Source: CAD feature listing. Evaluate the final solid. Frame: model axes, mm. A direction names the side the tool comes from. Give positions to 0.01 mm unless a question says otherwise; leave off trailing zeros. Loops run counter-clockwise (first coordinate to the right, second up) from the corner with the lowest first, then second, coordinate; pieces in that order, holes last. Notation, with made-up numbers: (8.25, -32) - (67.25, -32) arc R23 cw to (67.25, -14) - close; hole circle Ø5 at (79, -24). An arc over 180 degrees is marked (long way). Write each question's results on one line, items separated by ' | '. Start each with the question number.
(1) Reachability of faces 1 (the cylindrical face through (0.333, -1.463, 2.535)), 2 (the flat face through (0, 0, 5)) from +Z, -Z, +X, -X, +Y, -Y: full face, straight path, thin tool, end or side. Return the list, or none.
(2) Cut plane D-D on x = 0.25. Return the cut outline in (y, z), then the cut area to 3 significant figures.
(3) Cut plane C-C on x = 2.5. Return the cut outline in (y, z), then the cut area to 3 significant figures.
(4) Contact query for flat-ended pins moving along their axis: pin 1 (2 mm diameter, centred on x = 1.5, z = 2, fed in from -Y); pin 2 (3 mm diameter, centred on y = 3.5, z = 1.5, fed in from +X); pin 3 (2 mm diameter, centred on x = 5, z = 0.5, fed in from -Y). Output: stop coordinate, or through.
(5) Material intervals for line 1 along X through (y, z) = (-4, 3.2); line 2 along X through (y, z) = (4, 3.7); line 3 along Y through (x, z) = (-4.5, 2.35), sorted ascending. Write a range as [from, to].
(6) Cut plane B-B on y = -1.75. Return the cut outline in (x, z), then the cut area to 3 significant figures.
(7) Cut plane A-A on z = 0.45. Return the cut outline in (x, y).
(8) Pull-direction query (Y, two-part tool) for faces 3 (the flat face through (0, 0, 0)), 4 (the cylindrical face through (-1.46, -6.59, 2.46)), 5 (the flat face through (0, 4, 3)); classes: pulls with the +Y half, pulls with the -Y half, needs draft (parallel to the pull), parting line crosses it, or undercut.
from build123d import *

# Parameters (mm, degrees)
F0_R     = 6.75
F1_DEPTH = 5
F3_DEPTH = 25


# Not quite as in the source:
# - a feature names something its author has since deleted; it is built from what else it names


with BuildPart() as f1:
    # F0 (on Top) → F1 (new body)
    with BuildSketch(Plane.XY):
        Circle(F0_R)
    extrude(amount=F1_DEPTH)

    # F2 (on face) → F3 (cut)
    with BuildSketch(Plane.XY.offset(5)):
        with BuildLine():
            Line((1.0970305524, 1.0229975401), (4.02115299, 3.7497858268))
            ThreePointArc((4.02115299, 3.7497858268), (2.192415253, 5.04220988), (0, 5.4982329084))
            Line((0, 5.4982329084), (0, 1.5))
            ThreePointArc((0, 1.5), (0.5981236034, 1.3755901116), (1.0970305524, 1.0229975401))
        make_face()
        with BuildLine():
            Line((-0.6339273926, 1.3594616806), (-2.3236536344, 4.9830912999))
            ThreePointArc((-2.3236536344, 4.9830912999), (-4.117932991, 3.6432393549), (-5.2291302357, 1.6990474077))
            Line((-5.2291302357, 1.6990474077), (-1.4265847744, 0.4635254916))
            ThreePointArc((-1.4265847744, 0.4635254916), (-1.1234335812, 0.9939300723), (-0.6339273926, 1.3594616806))
        make_face()
        with BuildLine():
            ThreePointArc((-5.4572499141, -0.6700660344), (-4.7374378048, -2.7905641295), (-3.2317802172, -4.448163862))
            Line((-3.2317802172, -4.448163862), (-0.8816778784, -1.2135254916))
            ThreePointArc((-0.8816778784, -1.2135254916), (-1.2924437407, -0.7613075444), (-1.4888192275, -0.1828040151))
            Line((-1.4888192275, -0.1828040151), (-5.4572499141, -0.6700660344))
        make_face()
        with BuildLine():
            ThreePointArc((-1.0491122976, -5.3972148839), (1.190035408, -5.3679028347), (3.2317802172, -4.448163862))
            Line((3.2317802172, -4.448163862), (0.8816778784, -1.2135254916))
            ThreePointArc((0.8816778784, -1.2135254916), (0.3246594209, -1.4644440107), (-0.2862134931, -1.4724407752))
            Line((-0.2862134931, -1.4724407752), (-1.0491122976, -5.3972148839))
        make_face()
        with BuildLine():
            ThreePointArc((4.8088628562, -2.6655962084), (5.3231012166, -1.3766475779), (5.4982329084, 0))
            ThreePointArc((5.4982329084, 0), (5.4305405375, 0.8601131237), (5.2291302357, 1.6990474077))
            Line((5.2291302357, 1.6990474077), (1.4265847744, 0.4635254916))
            ThreePointArc((1.4265847744, 0.4635254916), (1.4815325109, 0.2346516976), (1.5, 0))
            ThreePointArc((1.5, 0), (1.4522214606, -0.3755700061), (1.3119295607, -0.7272144304))
            Line((1.3119295607, -0.7272144304), (4.8088628562, -2.6655962084))
        make_face()
    extrude(amount=-F3_DEPTH, mode=Mode.SUBTRACT)


solid = f1.part
Ans:
1) face 1: +Z, -Z | face 2: +Z, +X, -X, +Y, -Y
2) outline: (-6.75, 0) - (-5.49, 0) - (-5.49, 5) - (-6.75, 5) - close; (-1.48, 0) - (1.48, 0) - (1.48, 5) - (-1.48, 5) - close; (5.49, 0) - (6.75, 0) - (6.75, 5) - (5.49, 5) - close | area: 27.3 mm^2
3) outline: (-6.27, 0) - (-4.9, 0) - (-4.9, 5) - (-6.27, 5) - close; (-3.44, 0) - (-1.39, 0) - (-1.39, 5) - (-3.44, 5) - close; (0.81, 0) - (2.33, 0) - (2.33, 5) - (0.81, 5) - close; (4.9, 0) - (6.27, 0) - (6.27, 5) - (4.9, 5) - close | area: 31.6 mm^2
4) pin 1: y = -6.73 | pin 2: x = 6.45 | pin 3: y = -5.44
5) line 1: [-5.44, -3.77], [-2.91, -0.78], [2.91, 5.44] | line 2: [-5.44, -3.77], [-1.87, 0], [3.77, 5.44] | line 3: [-5.03, -3.16], [-0.55, 1.46], [3.16, 5.03]
6) outline: (-6.52, 0) - (-5.21, 0) - (-5.21, 5) - (-6.52, 5) - close; (-1.27, 0) - (-0.34, 0) - (-0.34, 5) - (-1.27, 5) - close; (1.27, 0) - (3.16, 0) - (3.16, 5) - (1.27, 5) - close; (5.21, 0) - (6.52, 0) - (6.52, 5) - (5.21, 5) - close | area: 27.2 mm^2
7) outline: circle Ø13.5 at (0, 0); hole (-5.46, -0.67) arc R5.5 ccw to (-3.23, -4.45) - (-0.88, -1.21) arc R1.5 cw to (-1.49, -0.18) - close; hole (-5.23, 1.7) - (-1.43, 0.46) arc R1.5 cw to (-0.63, 1.36) - (-2.32, 4.98) arc R5.5 ccw to start; hole (-1.05, -5.4) arc R5.5 ccw to (3.23, -4.45) - (0.88, -1.21) arc R1.5 cw to (-0.29, -1.47) - close; hole (0, 1.5) arc R1.5 cw to (1.1, 1.02) - (4.02, 3.75) arc R5.5 ccw to (0, 5.5) - close; hole (1.31, -0.73) - (4.81, -2.67) arc R5.5 ccw to (5.23, 1.7) - (1.43, 0.46) arc R1.5 cw to start
8) face 3: needs draft | face 4: parting line crosses it | face 5: undercut
